Geometry check sheet. Reference: drawing and pictorial views, mm from the part's lowest x, y, z. A direction names the side the tool comes from. Give positions to 0.01 mm unless a question says otherwise; leave off trailing zeros. Order: outer loops, then holes, each group sorted by start corner. A loop starts at its lowest first (then second) coordinate and runs counter-clockwise, first axis right, second up.
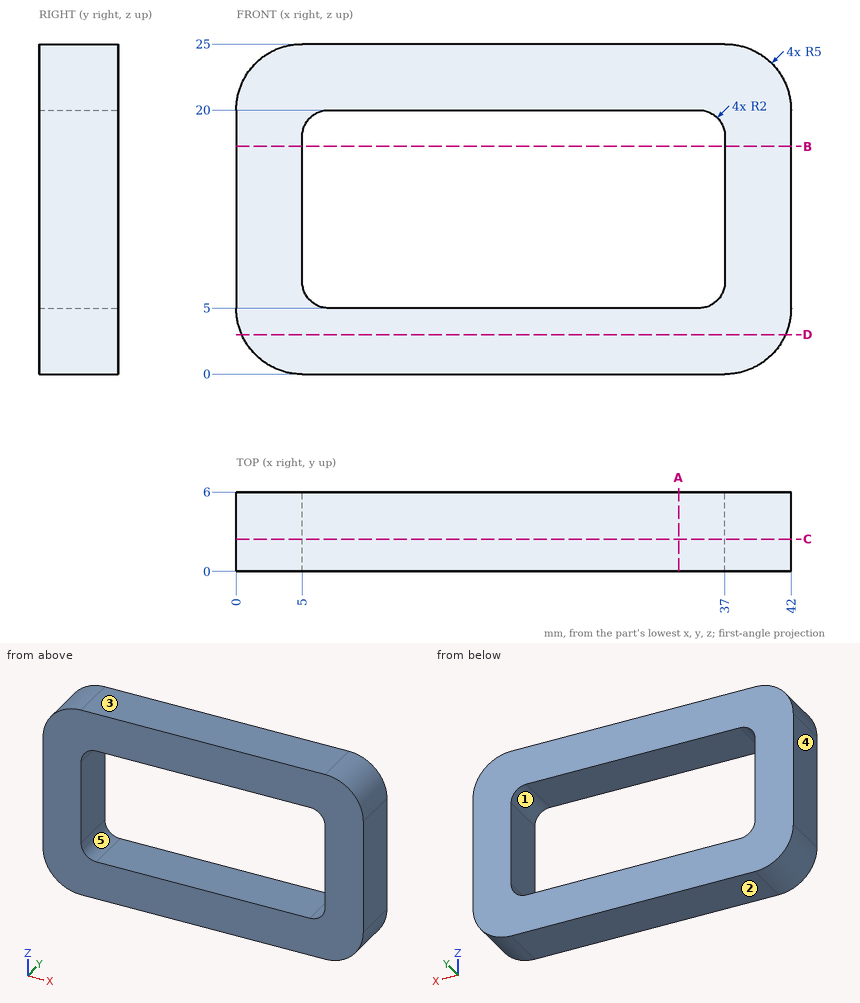
1) Draft check along Z on the marked faces 1, 2 and 3. Enter one of: +Z half, -Z half, draft (parallel to the pull), parting line (faces both ways), or undercut.
Recorded:
face 1: undercut
face 2: -Z half
face 3: +Z half
2) Section check C-C, the plane y = 2.45. Record the cut outline in (x, z), then the cut area to 3 significant figures.
Recorded:
outline: (0, 5) arc R5 ccw to (5, 0) - (37, 0) arc R5 ccw to (42, 5) - (42, 20) arc R5 ccw to (37, 25) - (5, 25) arc R5 ccw to (0, 20) - close; hole (5, 7) arc R2 ccw to (7, 5) - (35, 5) arc R2 ccw to (37, 7) - (37, 18) arc R2 ccw to (35, 20) - (7, 20) arc R2 ccw to (5, 18) - close
area: 552 mm2
3) Set-up check for the marked faces 4 and 5: record each of +Z, -Z, +X, -X, +Y, -Y from which the full face is reachable in a straight line by a thin tool's end or side.
Recorded:
face 4: +Z, -Z, -X, +Y, -Y
face 5: +Y, -Y
4) Material ranges on L1, parallel to Z at x = 10.5, y = 1.65; L2, parallel to X at y = 1.25, z = 9; L3, parallel to Z at x = 6, y = 2.7, recorded low to high.
Recorded:
L1: z = 0 to 5, 20 to 25
L2: x = 0 to 5, 37 to 42
L3: z = 0 to 5.27, 19.73 to 25
5) Depth check by flat-ended pin: pin 1 Ø8 at (x, z) = (18, 17) entering from -Y. Enter the tip coordinate at first touch or a pass-through.
Recorded:
pin 1: stops at y = 0
6) Section check B-B, the plane z = 17.25. Record the cut outline in (x, y).
Recorded:
outline: (0, 0) - (5, 0) - (5, 6) - (0, 6) - close; (37, 0) - (42, 0) - (42, 6) - (37, 6) - close
7) Section check D-D, the plane z = 3. Record the cut outline in (x, y), then the cut area to 3 significant figures.
Recorded:
outline: (0.42, 0) - (41.58, 0) - (41.58, 6) - (0.42, 6) - close
area: 247 mm2
8) Section check A-A, the plane x = 33.5. Record the cut outline in (y, z), then the cut area to 3 significant figures.
Recorded:
outline: (0, 0) - (6, 0) - (6, 5) - (0, 5) - close; (0, 20) - (6, 20) - (6, 25) - (0, 25) - close
area: 60.0 mm2
